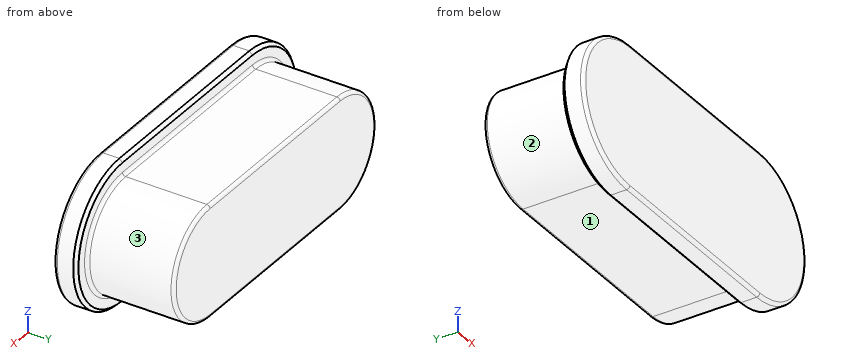
from build123d import *

# Parameters (mm, degrees)
BOSS_EXTRU_1_DEPTH = 0.7
BOSS_EXTRU_2_DEPTH = 2.75
CONG_1_R           = 0.1
CONG_2_R           = 0.1
CONG_3_R           = 0.1
CHANFREIN1_SIZE    = 0.1


with BuildPart() as part:
    # Esquisse1 → Boss.-Extru.1 (new body)
    with BuildSketch(Plane(origin=(0, 0, 0), x_dir=(1, 0, 0), z_dir=(0, 1, 0))):
        with BuildLine():
            Line((0, 2.25), (6.35, 2.25))
            ThreePointArc((6.35, 2.25), (8.6, 0), (6.35, -2.25))
            Line((6.35, -2.25), (0, -2.25))
            ThreePointArc((0, -2.25), (-2.25, 0), (0, 2.25))
        make_face()
    extrude(amount=BOSS_EXTRU_1_DEPTH)

    # Esquisse2 → Boss.-Extru.2 (add)
    with BuildSketch(Plane(origin=(0, 0.7, 0), x_dir=(1, 0, 0), z_dir=(0, 1, 0))):
        with BuildLine():
            Line((0, 1.75), (6.35, 1.75))
            ThreePointArc((6.35, 1.75), (8.1, 0), (6.35, -1.75))
            Line((6.35, -1.75), (0, -1.75))
            ThreePointArc((0, -1.75), (-1.75, 0), (0, 1.75))
        make_face()
    extrude(amount=BOSS_EXTRU_2_DEPTH)

    # Congé1
    cong_1_edges = [part.edges().sort_by_distance(p)[0] for p in [
        (-1.75, 0.7, 0),
        (3.175, 0.7, 1.75),
        (8.1, 0.7, 0),
        (3.175, 0.7, -1.75),
    ]]
    fillet(cong_1_edges, radius=CONG_1_R)

    # Congé2
    cong_2_edges = [part.edges().sort_by_distance(p)[0] for p in [
        (-1.75, 3.45, 0),
        (3.175, 3.45, 1.75),
        (8.1, 3.45, 0),
        (3.175, 3.45, -1.75),
    ]]
    fillet(cong_2_edges, radius=CONG_2_R)

    # Congé3
    cong_3_edges = [part.edges().sort_by_distance(p)[0] for p in [
        (3.175, 0, -2.25),
        (8.6, 0, 0),
        (3.175, 0, 2.25),
        (-2.25, 0, 0),
    ]]
    fillet(cong_3_edges, radius=CONG_3_R)

    # Chanfrein1
    chanfrein1_edges = [part.edges().sort_by_distance(p)[0] for p in [
        (8.6, 0.7, 0),
        (3.175, 0.7, -2.25),
        (-2.25, 0.7, 0),
        (3.175, 0.7, 2.25),
    ]]
    chamfer(chanfrein1_edges, length=CHANFREIN1_SIZE)


solid = part.part
Build history of the part. All positions in model axes, mm. Face numbers are marked on the shaded views. A direction names the side the tool comes from. Round coordinates to 2 decimals unless told otherwise and drop trailing zeros. Loops run counter-clockwise (first coordinate to the right, second up) from the corner with the lowest first, then second, coordinate; pieces in that order, holes last. Notation, with made-up numbers: (4, 16) -> (12, 16) arc R23 cw to (12, 28) -> close; hole circle Ø7 at (68.5, 36.5). An arc over 180 degrees is marked (long way). Use CSV: the item, a comma, the result in double quotes. Start each with the question number.
Q1. Flat gauge pins, fed straight in: pin 1 Ø1 at (x, y) = (4.5, 2) entering from -Z; pin 2 Ø1 at (x, y) = (-0.5, 2) entering from -Z; pin 3 Ø1.3 at (x, y) = (2, 2.5) entering from +Z. Where does each tip first touch, or does it go through?
Q2. Saw through at B-B on z = 0. Give the cut face in (x, y).
Q3. Saw through at A-A on x = 5.5. Give the cut face in (y, z).
Q4. Drill centre lines: L1, parallel to Y at x = 7.5, z = -1.55; L2, parallel to Z at x = 1.5, y = 3.1; L3, parallel to X at y = 1.1, z = 1.3. Where is each one in solid material? Low to high.
Q5. Which spindle directions (+Z, -Z, +X, -X, +Y, -Y) get a long thin tool onto all of the face, cutting with end or side? Do the marked faces 1, 2 and 3. Say none if no direction does.
Q6. Saw through at C-C on y = 1.2. Give the cut face in (x, z).
Solutions:
1,pin 1,"stops at z = -1.75"
1,pin 2,"stops at z = -1.75"
1,pin 3,"stops at z = 1.75"
2,outline,"(-2.25, 0.1) arc R0.1 ccw to (-2.15, 0) -> (8.5, 0) arc R0.1 ccw to (8.6, 0.1) -> (8.6, 0.6) -> (8.5, 0.7) -> (8.2, 0.7) arc R0.1 cw to (8.1, 0.8) -> (8.1, 3.35) arc R0.1 ccw to (8, 3.45) -> (-1.65, 3.45) arc R0.1 ccw to (-1.75, 3.35) -> (-1.75, 0.8) arc R0.1 cw to (-1.85, 0.7) -> (-2.15, 0.7) -> (-2.25, 0.6) -> close"
3,outline,"(0, -2.15) arc R0.1 ccw to (0.1, -2.25) -> (0.6, -2.25) -> (0.7, -2.15) -> (0.7, -1.85) arc R0.1 cw to (0.8, -1.75) -> (3.35, -1.75) arc R0.1 ccw to (3.45, -1.65) -> (3.45, 1.65) arc R0.1 ccw to (3.35, 1.75) -> (0.8, 1.75) arc R0.1 cw to (0.7, 1.85) -> (0.7, 2.15) -> (0.6, 2.25) -> (0.1, 2.25) arc R0.1 ccw to (0, 2.15) -> close"
4,L1,"y = 0 to 0.7"
4,L2,"z = -1.75 to 1.75"
4,L3,"x = -1.17 to 7.52"
5,face 1,"-Z, +X, -X, +Y"
5,face 2,"-X, +Y"
5,face 3,"+X, +Y"
6,outline,"(0, -1.75) -> (6.35, -1.75) arc R1.75 ccw to (6.35, 1.75) -> (0, 1.75) arc R1.75 ccw to start"
